Geometry: final body of the model. Coordinates: model frame, mm. Face numbers are marked on the shaded views. Round coordinates to 2 decimals unless told otherwise and drop trailing zeros. Loops run counter-clockwise (first coordinate to the right, second up) from the corner with the lowest first, then second, coordinate; pieces in that order, holes last. Notation, with made-up numbers: M -12,1 L 22,1 A27 cw 22,25 Z; hole C 9,-18.5 d10. An arc over 180 degrees is marked long. Return JSON: item names as keys, results as strings.
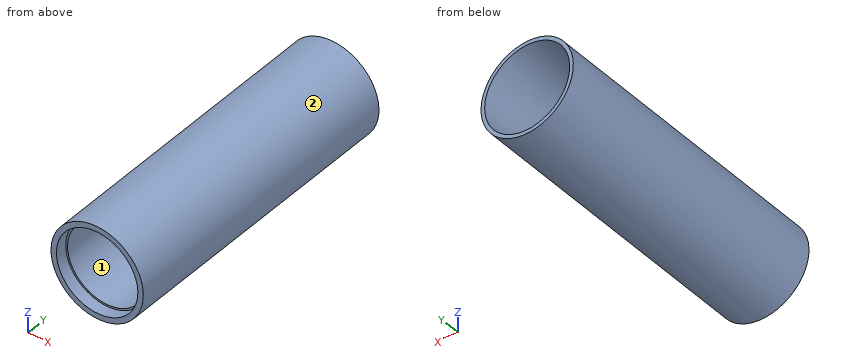
from build123d import *

# Parameters (mm, degrees)
SKETCH1_R           = 12.7
BOSS_EXTRUDE1_DEPTH = 82
SKETCH2_R           = 11.7
CUT_EXTRUDE1_DEPTH  = 25.4
CUT_EXTRUDE1_DRAFT  = -5
SKETCH3_R           = 10.7
CUT_EXTRUDE2_DEPTH  = 53.38
SKETCH4_R           = 11.2
CUT_EXTRUDE3_DEPTH  = 81.801413354


with BuildPart() as part:
    # Sketch1 → Boss-Extrude1 (new body)
    with BuildSketch(Plane(origin=(0, 0, 0), x_dir=(1, 0, 0), z_dir=(0, 1, 0))):
        with Locations(Location((0, 0, 0), (0, 0, 270))):
            Circle(SKETCH1_R)
    extrude(amount=-BOSS_EXTRUDE1_DEPTH)


with BuildPart() as cut_extrude1_tool:
    # Sketch2 → Cut-Extrude1 (with draft: the straight prism first)
    with BuildSketch(Plane(origin=(0, 0, 0), x_dir=(1, 0, 0), z_dir=(0, 1, 0))):
        Circle(SKETCH2_R)
    extrude(amount=-CUT_EXTRUDE1_DEPTH)
    # Cut-Extrude1: the draft: its side faces are tilted about the plane it starts from
    cut_extrude1_sides = [cut_extrude1_tool.faces().sort_by_distance(p)[0] for p in [
        (-11.7, -12.7, 0),
    ]]
    draft(cut_extrude1_sides, Plane(origin=(0, 0, 0), x_dir=(1, 0, 0), z_dir=(0, 1, 0)), CUT_EXTRUDE1_DRAFT)


with BuildPart() as part_1:
    add(part.part)

    # Cut-Extrude1: cut by cut_extrude1_tool
    add(cut_extrude1_tool.part, mode=Mode.SUBTRACT)

    # Sketch3 → Cut-Extrude2 (cut)
    with BuildSketch(Plane(origin=(0, -25.4, 0), x_dir=(1, 0, 0), z_dir=(0, 1, 0))):
        with Locations(Location((0, 0, 0), (0, 0, 270))):
            Circle(SKETCH3_R)
    extrude(amount=-CUT_EXTRUDE2_DEPTH, mode=Mode.SUBTRACT)

    # Sketch4 → Cut-Extrude3 (cut, through all)
    with BuildSketch(Plane(origin=(0, -78.78, 0), x_dir=(1, 0, 0), z_dir=(0, 1, 0))):
        with Locations(Location((0, 0, 0), (0, 0, 270))):
            Circle(SKETCH4_R)
    extrude(amount=-CUT_EXTRUDE3_DEPTH, mode=Mode.SUBTRACT)


solid = part_1.part
Q1. Pin query (flat end, axial travel): pin 1 (11 mm diameter, centred on x = -0.5, z = 0, fed in from -Y); pin 2 (3 mm diameter, centred on x = 7, z = 6.5, fed in from -Y); pin 3 (6 mm diameter, centred on x = -9, y = -21, fed in from +Z); pin 4 (8 mm diameter, centred on x = -8.5, y = -31.5, fed in from +Z). Return the tip coordinate at first contact, or that it passes through.
Determined:
{"pin 1": "passes through", "pin 2": "stops at y = -78.78", "pin 3": "stops at z = 11.19", "pin 4": "stops at z = 11.88"}
Q2. Section query C-C (y = -27). Output: boundary loops of the cut face in (x, z), plus the area to 3 significant figures.
Determined:
{"outline": "C 0,0 d25.4; hole C 0,0 d21.4", "area": "147 mm^2"}
Q3. Pull-direction query (Z, two-part tool) for the marked faces 1 and 2; classes: pulls with the +Z half, pulls with the -Z half, needs draft (parallel to the pull), parting line crosses it, or undercut.
Determined:
{"face 1": "undercut", "face 2": "parting line crosses it"}
Q4. Section query A-A (x = 0). Output: boundary loops of the cut face in (y, z).
Determined:
{"outline": "M -82,-12.7 L 0,-12.7 L 0,-11.7 L -25.4,-9.48 L -25.4,-10.7 L -78.78,-10.7 L -78.78,-11.2 L -82,-11.2 Z; M -82,11.2 L -78.78,11.2 L -78.78,10.7 L -25.4,10.7 L -25.4,9.48 L 0,11.7 L 0,12.7 L -82,12.7 Z"}
Q5. Section query B-B (z = 0). Output: boundary loops of the cut face in (x, y).
Determined:
{"outline": "M -12.7,-82 L -11.2,-82 L -11.2,-78.78 L -10.7,-78.78 L -10.7,-25.4 L -9.48,-25.4 L -11.7,0 L -12.7,0 Z; M 9.48,-25.4 L 10.7,-25.4 L 10.7,-78.78 L 11.2,-78.78 L 11.2,-82 L 12.7,-82 L 12.7,0 L 11.7,0 Z"}
Q6. Material intervals for L1, parallel to X at y = -80.7, z = 0; L2, parallel to X at y = -45, z = 0; L3, parallel to Z at x = -9.75, y = -61.5, sorted ascending.
Determined:
{"L1": "x = -12.7 to -11.2, 11.2 to 12.7", "L2": "x = -12.7 to -10.7, 10.7 to 12.7", "L3": "z = -8.14 to -4.41, 4.41 to 8.14"}
